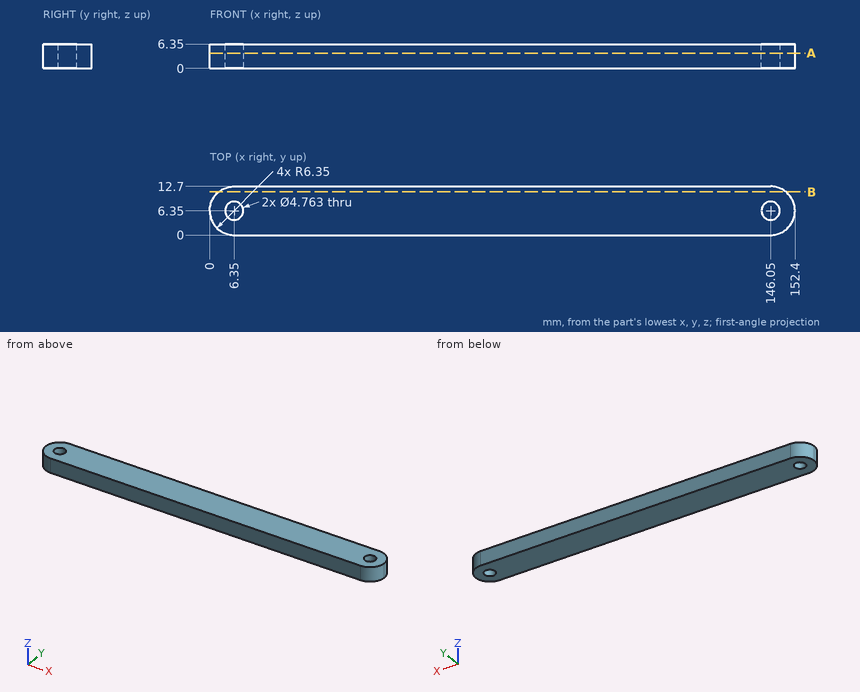
Geometry check sheet. Reference: drawing and pictorial views, mm from the part's lowest x, y, z. Coordinates: 2 decimals unless noted, no trailing zeros. Order: outer loops, then holes, each group sorted by start corner. A loop starts at its lowest first (then second) coordinate and runs counter-clockwise, first axis right, second up. Notation, with made-up numbers: (-15, 46) -> (38, 46) arc R32 cw to (38, 77) -> close; hole circle Ø7 at (-14, 11). An arc over 180 degrees is marked (long way). Put each result on its own line as item: value. Start each with the question number.
1) Cross-section at A-A (z = 4). State how many separate pieces and enclosed holes the cut face has.
2) Cross-section at B-B (y = 11.25). Enter the section's corners in (x, z).
3) Material ranges on L1, parallel to Y at x = 146.05, z = 3.25; L2, parallel to X at y = 7.5, z = 3.25 (1 decimal); L3, parallel to X at y = 5.5, z = 1.75 (1 decimal), recorded low to high.
Geometry check:
1. separate pieces: 1
1. enclosed holes: 2
2. outline: (2.31, 0) -> (150.09, 0) -> (150.09, 6.35) -> (2.31, 6.35) -> close
3. L1: y = 0 to 3.97, 8.73 to 12.7
3. L2: x = 0.1 to 4.3, 8.4 to 144, 148.1 to 152.3
3. L3: x = 0.1 to 4.1, 8.6 to 143.8, 148.3 to 152.3
